```python
from build123d import *

# Parameters (mm, degrees)
SKETCH1_R           = 1.65
BOSS_EXTRUDE3_DEPTH = 3
CUT_EXTRUDE1_DEPTH  = 4
SKETCH4_R           = 1.75
CUT_EXTRUDE2_DEPTH  = 4
SKETCH5_R           = 10
CUT_EXTRUDE3_DEPTH  = 4
FILLET1_R           = 2.54


with BuildPart() as part:
    # Sketch1 → Boss-Extrude3 (new body)
    with BuildSketch(Plane(origin=(0, 0, 0), x_dir=(1, 0, 0), z_dir=(0, 1, 0))):
        with BuildLine():
            Line((48.284490735, 53.109977813), (-64.735509285, 53.109977813))
            Line((-64.735509285, 53.109977813), (-64.735509285, -72.290076187))
            Line((-64.735509285, -72.290076187), (22.884490735, -72.290076187))
            ThreePointArc((22.884490735, -72.290076187), (40.845002977, -64.850588429), (48.284490735, -46.890076187))
            Line((48.284490735, -46.890076187), (48.284490735, 53.109977813))
        make_face()
        with Locations((-59.655509285, 48.029977813)):
            Circle(SKETCH1_R, mode=Mode.SUBTRACT)
        with Locations((43.204490735, 48.029977813)):
            Circle(SKETCH1_R, mode=Mode.SUBTRACT)
        with Locations((-59.655509285, -67.210076187)):
            Circle(SKETCH1_R, mode=Mode.SUBTRACT)
        with Locations((37.880892571, -60.748479124)):
            Circle(SKETCH1_R, mode=Mode.SUBTRACT)
    extrude(amount=BOSS_EXTRUDE3_DEPTH)

    # Sketch3 → Cut-Extrude1 (cut, through all)
    with BuildSketch(Plane(origin=(0, 3, 0), x_dir=(1, 0, 0), z_dir=(0, 1, 0))):
        with BuildLine():
            Line((-10.308309275, 24.029977813), (-10.308309275, 21.220282526))
            ThreePointArc((-10.308309275, 21.220282526), (-8.225509275, 14.219977813), (-6.142709275, 21.220282526))
            Line((-6.142709275, 21.220282526), (-6.142709275, 24.029977813))
            ThreePointArc((-6.142709275, 24.029977813), (-8.225509275, 26.112777813), (-10.308309275, 24.029977813))
        make_face()
    extrude(amount=-CUT_EXTRUDE1_DEPTH, mode=Mode.SUBTRACT)

    # Sketch4 → Cut-Extrude2 (cut, through all)
    with BuildSketch(Plane(origin=(0, 3, 0), x_dir=(1, 0, 0), z_dir=(0, 1, 0))):
        with Locations((-49.935509285, -6.820022187)):
            Circle(SKETCH4_R)
        with Locations((-6.755509285, -41.110022187)):
            Circle(SKETCH4_R)
        with Locations((-10.565509285, 33.819977813)):
            Circle(SKETCH4_R)
    extrude(amount=-CUT_EXTRUDE2_DEPTH, mode=Mode.SUBTRACT)

    # Sketch5 → Cut-Extrude3 (cut, through all)
    with BuildSketch(Plane(origin=(0, 3, 0), x_dir=(1, 0, 0), z_dir=(0, 1, 0))):
        with Locations((-8.225509275, -9.590049187)):
            Circle(SKETCH5_R)
    extrude(amount=-CUT_EXTRUDE3_DEPTH, mode=Mode.SUBTRACT)

    # Fillet1
    fillet1_edges = [part.edges().sort_by_distance(p)[0] for p in [
        (-64.735509285, 1.5, 72.290076187),
        (-64.735509285, 1.5, -53.109977813),
        (48.284490735, 1.5, -53.109977813),
    ]]
    fillet(fillet1_edges, radius=FILLET1_R)


solid = part.part
```
Part model, mm, in its own coordinate system. A direction names the side the tool comes from. Give positions to 0.01 mm unless a question says otherwise; leave off trailing zeros. Write each loop counter-clockwise with the first axis right and the second up, starting at its lowest first coordinate (ties: lowest second). Pieces come first, ordered by that corner, then holes. Notation, with made-up numbers: (83.5, 48) -> (115.5, 48) arc R19 ccw to (115.5, 56) -> close; hole circle Ø4 at (47, 16.25). An arc over 180 degrees is marked (long way). Put each result on its own line as item: value. Start each with the question number.
Item 1: Cut at C-C (x = -16.5). List the corners of the cut face in (y, z), then the cut area to 3 significant figures.
Item 2: Cut at B-B (y = 2). State how many separate pieces and enclosed holes the cut face has, then the cut area to 3 significant figures.
Item 3: Which spindle directions (+Z, -Z, +X, -X, +Y, -Y) get a long thin tool onto all of the face, cutting with end or side? Do faces 4 (the face through (48.284, 1, -1)), 5 (the face through (-10.308, 2, -23)). Say none if no direction does.
Item 4: Pull direction Z, two halves, no side cores. Call faces 1 (the face through (4, 3, 9)), 2 (the face through (-48.266, 1.521, 6.294)), 3 (the face through (40.646, 1.479, 65.047)): pulls with the +Z half, pulls with the -Z half, needs draft (parallel to the pull), parting line crosses it, or undercut.
Item 5: Pin check, flat tip, straight feed: pin 1 Ø12 at (x, z) = (-8.23, 9.59) entering from +Y. Stop position of the tip, or through.
Item 6: Wall check: L1, parallel to Z at x = 39, y = 2.6; L2, parallel to Z at x = -58.5, y = 1.45; L3, parallel to Z at x = 1, y = 0.4. Give the ranges that are in metal, low to high. Write a range as [from, to].
Item 7: Cut at A-A (z = -16). List the corners of the cut face in (x, y), then the cut area to 3 significant figures.
Answer list:
1. outline: (0, -53.11) -> (3, -53.11) -> (3, 3.97) -> (0, 3.97) -> close; (0, 15.21) -> (3, 15.21) -> (3, 72.29) -> (0, 72.29) -> close
1. area: 343 mm2
2. separate pieces: 1
2. enclosed holes: 9
2. area: 13,600 mm2
3. face 4: +Z, -Z, +X, +Y, -Y
3. face 5: +Y, -Y
4. face 1: needs draft
4. face 2: undercut
4. face 3: pulls with the +Z half
5. pin 1: passes through
6. L1: z = [-53.11, 59.54], [61.96, 66.52]
6. L2: z = [-53.11, -49.21], [-46.85, 66.03], [68.39, 72.29]
6. L3: z = [-53.11, 5.73], [13.45, 72.29]
7. outline: (-64.74, 0) -> (-11.45, 0) -> (-11.45, 3) -> (-64.74, 3) -> close; (-5, 0) -> (48.28, 0) -> (48.28, 3) -> (-5, 3) -> close
7. area: 320 mm2
